from build123d import *
from build123d.topology import SkipClean

# Parameters (mm, degrees)
MAIN_PROFILE_W     = 10
MAIN_PROFILE_H     = 0.8
CLAMP_CUTOFF_ANGLE = 15
CLAMP_BODY_ANGLE   = 14
CLAMP_ARRAY_COUNT  = 4
HOLES_ARRAY_COUNT  = 4


with BuildPart() as part:
    # Main_profile → Main_body (revolve)
    with BuildSketch(Plane(origin=(0, 0, 0), x_dir=(1, 0, 0), z_dir=(0, 1, 0)), mode=Mode.PRIVATE) as main_body_sk:
        Polygon((-75, 1.2), (-74.159750954, 0), (-62.45, 0), (-62.45, 0.8), (-52.45, 0.8), (-55.629352876, 17.4), (-59.333436307, 17.4), (-59.933436307, 5.054759753), (-60.333436307, 5.054759753), (-62.333436307, 5.054759753), (-62.5, 1.2), align=None)
        with Locations((-57.45, 0.4)):
            Rectangle(MAIN_PROFILE_W, MAIN_PROFILE_H)
        Polygon((-60.333436307, 17.4), (-60.333436307, 5.054759753), (-59.933436307, 5.054759753), (-59.333436307, 17.4), align=None)
        Polygon((-62.307188758, 5.662203024), (-62.333436307, 5.054759753), (-60.333436307, 5.054759753), (-60.333436307, 17.4), (-61.50694686, 17.4), (-61.844316804, 16.37438253), align=None)
        Polygon((-61.8, 17.4), (-61.844316804, 16.37438253), (-61.50694686, 17.4), align=None)
        with Locations((-57.45, 0.4)):
            Rectangle(MAIN_PROFILE_W, MAIN_PROFILE_H)
    revolve(main_body_sk.sketch.rotate(Axis((0, 0, 21.596985385), (0, 0, -1)), 180), axis=Axis((0, 0, 21.596985385), (0, 0, -1)))

    # Sketch 1_8 → clamp_cutoff (revolve, symmetric, cut)
    with BuildSketch(Plane(origin=(0, 0, 0), x_dir=(1, 0, 0), z_dir=(0, 1, 0))) as clamp_cutoff_sk:
        Polygon((-60.333436307, 17.4), (-60.333436307, 5.054759753), (-59.933436307, 5.054759753), (-59.333436307, 17.4), align=None)
        Polygon((-62.307188758, 5.662203024), (-62.333436307, 5.054759753), (-60.333436307, 5.054759753), (-60.333436307, 17.4), (-61.50694686, 17.4), (-61.844316804, 16.37438253), align=None)
        Polygon((-61.8, 17.4), (-61.844316804, 16.37438253), (-61.50694686, 17.4), align=None)
    clamp_cutoff = revolve(axis=Axis((0, 0, 21.596985385), (0, 0, -1)), revolution_arc=CLAMP_CUTOFF_ANGLE / 2, mode=Mode.SUBTRACT)
    clamp_cutoff = clamp_cutoff + revolve(clamp_cutoff_sk.sketch, axis=Axis((0, 0, 21.596985385), (0, 0, 1)), revolution_arc=CLAMP_CUTOFF_ANGLE / 2, mode=Mode.SUBTRACT)

    # Sketch 1_10 → Clamp_body (revolve, symmetric)
    with SkipClean():  # the faces are left unmerged after this step: merging them gives an invalid solid
        with BuildSketch(Plane(origin=(0, 0, 0), x_dir=(1, 0, 0), z_dir=(0, 1, 0))) as clamp_body_sk:
            Polygon((-62.307188758, 5.662203024), (-62.333436307, 5.054759753), (-60.333436307, 5.054759753), (-60.333436307, 17.4), (-61.50694686, 17.4), (-61.844316804, 16.37438253), align=None)
            Polygon((-62.7, 13.77307305), (-62.307188758, 5.662203024), (-61.844316804, 16.37438253), align=None)
        clamp_body = revolve(axis=Axis((0, 0, 21.596985385), (0, 0, -1)), revolution_arc=CLAMP_BODY_ANGLE / 2)
        clamp_body = clamp_body + revolve(clamp_body_sk.sketch, axis=Axis((0, 0, 21.596985385), (0, 0, 1)), revolution_arc=CLAMP_BODY_ANGLE / 2)

    # Clamp_array: clamp_cutoff, Clamp_body ×4 about axis
    with SkipClean():  # the faces are left unmerged after this step: merging them gives an invalid solid
        clamp_array_axis = Axis((0, 0, -17.4), (0, 0, 1))
        add([clamp_cutoff.rotate(clamp_array_axis, i * 360 / CLAMP_ARRAY_COUNT) for i in range(1, CLAMP_ARRAY_COUNT)], mode=Mode.SUBTRACT)
        add([clamp_body.rotate(clamp_array_axis, i * 360 / CLAMP_ARRAY_COUNT) for i in range(1, CLAMP_ARRAY_COUNT)])

    # Hole_profile → Hole (revolve, cut)
    with SkipClean():  # the faces are left unmerged after this step: merging them gives an invalid solid
        with BuildSketch(Plane(origin=(0, 0, 0), x_dir=(0, 0, -1), z_dir=(0.7071067811865488, 0.7071067811865464, 0)), mode=Mode.PRIVATE) as hole_sk:
            Polygon((0, 59.1), (0, 57.7), (15, 57.7), (13.441154273, 58.6), align=None)
        hole = revolve(hole_sk.sketch.rotate(Axis((-40.800061274, 40.800061274, 2.268978304), (0, 0, -1)), 135), axis=Axis((-40.800061274, 40.800061274, 2.268978304), (0, 0, -1)), mode=Mode.SUBTRACT)

    # Holes_array: Hole ×4 about axis
    with SkipClean():  # the faces are left unmerged after this step: merging them gives an invalid solid
        holes_array_axis = Axis((0, 0, 0), (0, 0, 1))
        for i in range(1, HOLES_ARRAY_COUNT):
            add(hole.rotate(holes_array_axis, i * 360 / HOLES_ARRAY_COUNT), mode=Mode.SUBTRACT)


solid = part.part
Input: part model. Units: mm. Frame: model coordinates. A direction names the side the tool comes from. Give positions to 0.01 mm unless a question says otherwise; leave off trailing zeros. Order: outer loops, then holes, each group sorted by start corner. A loop starts at its lowest first (then second) coordinate and runs counter-clockwise, first axis right, second up. Notation, with made-up numbers: (6.5, -6.5) - (62.5, -6.5) arc R33 cw to (62.5, 32.5) - close; hole circle Ø8 at (68, 53.5). An arc over 180 degrees is marked (long way). Answer as a JSON object with one key per item and string values. Group by question number.
Q1. Set-up query: faces 4 (the face through (0.103, -60.333, -11.314)), 5 (the face through (0.11, -62.5, -9.66)), 6 (the face through (-62.5, -0.11, -9.66)), 7 (the face through (15.4, -50.5, 0)). Return all of +Z, -Z, +X, -X, +Y, -Y with unobstructed straight access to the full face (end or side cutting, diameter ignored); none if empty.
Q2. Cut plane A-A, the plane z = -11.5. Count the separate pieces of the cut face and the enclosed holes in it, then the cut area to 3 significant figures.
Q3. Cut plane B-B, the plane z = -3.25. Output: boundary loops of the cut face in (x, y).
Q4. First-contact query: pin 1 Ø1 at (x, y) = (49.5, 14) entering from -Z; pin 2 Ø2.5 at (x, y) = (-60, -0.5) entering from -Z; pin 3 Ø1.5 at (x, z) = (-14, -3) entering from +Y; pin 4 Ø1.5 at (y, z) = (-53, -9) entering from -X. Flat tips, straight axial feed; report the tip coordinate or a pass-through.
Q5. Mould query, pull axis Y, two halves, no side actions, for faces 1 (the face through (-0.11, 62.5, -9.66)), 2 (the face through (-11.37, 51.203, -0.406)), 3 (the face through (62.5, 0.11, -9.66)). Classes: pulls with the +Y half, pulls with the -Y half, needs draft (parallel to the pull), parting line crosses it, or undercut.
Q6. Line query: probe 1 along X at (y, z) = (4.5, -16.5); probe 2 along Z at (x, y) = (-51, 49.5); probe 3 along X at (y, z) = (-6, -12.75). Output: solid intervals per line, ascending.
Results:
{
 "1": {"face 4": "-Z", "face 5": "-Y", "face 6": "-X", "face 7": "+Z, +X, -X, +Y, -Y"},
 "2": {"separate pieces": "5", "enclosed holes": "5", "area": "2,740 mm^2"},
 "3": {"outline": "circle Ø124.82 at (0, 0); hole circle Ø105.84 at (0, 0); hole circle Ø2.56 at (-40.8, -40.8); hole circle Ø2.56 at (-40.8, 40.8); hole circle Ø2.56 at (40.8, -40.8); hole circle Ø2.56 at (40.8, 40.8)"},
 "4": {"pin 1": "through", "pin 2": "z = -17.4", "pin 3": "y = 61", "pin 4": "x = -33.68"},
 "5": {"face 1": "pulls with the +Y half", "face 2": "undercut", "face 3": "parting line crosses it"},
 "6": {"probe 1": "-61.64 to -60.17, -59.21 to -55.27, 55.27 to 59.21, 60.17 to 61.64", "probe 2": "-1.2 to 0", "probe 3": "-62.36 to -60.03, -59.26 to -54.41, 54.41 to 59.26, 60.03 to 62.36"}
}
